Autodesk Inventor part; units mm, degrees
ref_plane "YZ Plane" through (0, 0, 0) normal (1, 0, 0) x (0, 1, 0)
ref_plane "XZ Plane" through (0, 0, 0) normal (0, 1, 0) x (-1, 0, 0)
ref_plane "XY Plane" through (0, 0, 0) normal (0, 0, 1) x (1, 0, 0)
sketch "Sketch1" plane through (0, 0, 0) normal (0, 0, 1) x (1, 0, 0)
  line L0 (2.6781, 6.36) -> (10.0219, 6.36)
  line L1 (-0.9939, 0) -> (2.6781, 6.36)
  line L2 (2.6781, -6.36) -> (-0.9939, 0)
  line L3 (10.0219, -6.36) -> (2.6781, -6.36)
  line L4 (13.6939, 0) -> (10.0219, -6.36)
  line L5 (10.0219, 6.36) -> (13.6939, 0)
  point P0 (0, 0)
extrude "Extrusion1" add sketch "Sketch1" along normal blind 457.2
properties part number "bigShaft2"
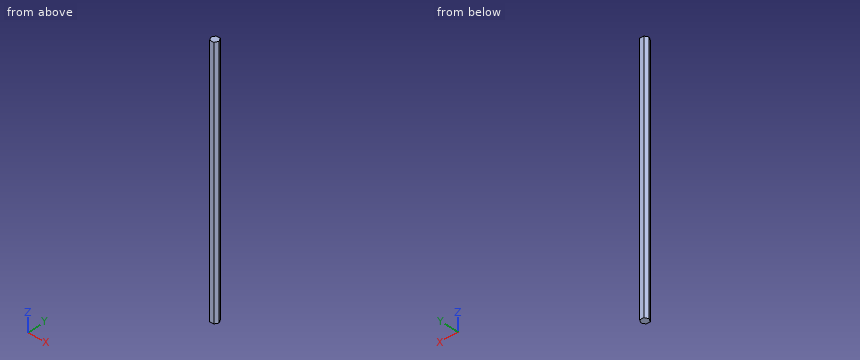
Here's how the part is built. I have some questions about the finished solid (model axes, mm). Give positions to 0.01 mm unless a question says otherwise; leave off trailing zeros. Order: outer loops, then holes, each group sorted by start corner. A loop starts at its lowest first (then second) coordinate and runs counter-clockwise, first axis right, second up. Notation, with made-up numbers: (-35, 40) -> (23, 40) arc R16 cw to (23, 49) -> close; hole circle Ø8 at (21.25, -9.75). An arc over 180 degrees is marked (long way). Use CSV: the item, a comma, the result in double quotes. Start each with the question number.
Item 1: I'm going to push a flat-ended pin straight in: P1, Ø6, axis at y = 3.5, z = 191.5, coming from the -X side. Where does the tip first touch, or does it pass through?
Item 2: Suppose I cut it at A-A (z = 140.5). List the corners of the cut face in (x, y) for me, and give its area (3 significant figures).
Item 3: Suppose I cut it at B-B (y = -3.5). List the corners of the cut face in (x, z) for me.
Item 4: If I drill on probe 1 along Y at (x, z) = (-0.5, 348.5); probe 2 along X at (y, z) = (6.25, 248); probe 3 along X at (y, z) = (5.75, 154), over which ranges is the centre line in solid material (lowest first)? Write a range as [from, to].
Answer block:
1,P1,"stops at x = -0.71"
2,outline,"(-0.99, 0) -> (2.68, -6.36) -> (10.02, -6.36) -> (13.69, 0) -> (10.02, 6.36) -> (2.68, 6.36) -> close"
2,area,"140 mm^2"
3,outline,"(1.03, 0) -> (11.67, 0) -> (11.67, 457.2) -> (1.03, 457.2) -> close"
4,probe 1,"y = [-0.86, 0.86]"
4,probe 2,"x = [2.61, 10.09]"
4,probe 3,"x = [2.33, 10.37]"
